Source: CAD feature listing. Evaluate the final solid. Frame: model axes, mm. Give positions to 0.01 mm unless a question says otherwise; leave off trailing zeros. Order: outer loops, then holes, each group sorted by start corner. A loop starts at its lowest first (then second) coordinate and runs counter-clockwise, first axis right, second up.
```python
from build123d import *

# Parameters (mm, degrees)
CYLINDER_R          = 3.4
CYLINDER_DEPTH      = 100
CYLINDER_ROLL_ANGLE = 90
SKETCH_R            = 11
PAD_DEPTH           = 30
SKETCH001_R         = 8.3
POCKET_DEPTH        = 30.001
CHAMFER_SIZE        = 0.5


with BuildPart() as cylinder:
    # Cylinder → Cylinder (new body)
    with BuildSketch(Plane.XY):
        Circle(CYLINDER_R)
    extrude(amount=CYLINDER_DEPTH)


with BuildPart() as cylinder_1:
    # Cylinder roll: moved
    add(cylinder.part.rotate(Axis((0, 0, 0), (1, 0, 0)), CYLINDER_ROLL_ANGLE))


with BuildPart() as cylinder_2:
    # Cylinder placement: moved
    add(cylinder_1.part.moved(Location((0, 16, 8.5))))


with BuildPart() as chamfer_body:
    # Sketch → Pad (new body)
    with BuildSketch(Plane.XY):
        Circle(SKETCH_R)
    extrude(amount=PAD_DEPTH)

    # Sketch001 → Pocket (cut, through all)
    with BuildSketch(Plane(origin=(0, 0, 0), x_dir=(1, 0, 0), z_dir=(0, 0, -1))):
        Circle(SKETCH001_R)
    extrude(amount=-POCKET_DEPTH, mode=Mode.SUBTRACT)

    # Cut: cut Cylinder
    add(cylinder_2.part, mode=Mode.SUBTRACT)

    # Chamfer
    chamfer_edges = [chamfer_body.edges().sort_by_distance(p)[0] for p in [
        (-8.3, 0, 0),
        (-8.3, 0, 30),
        (-11, 0, 30),
    ]]
    chamfer(chamfer_edges, length=CHAMFER_SIZE)


solid = chamfer_body.part
```
1) Section query A-A, the plane x = 0. Return the cut outline in (y, z), and give its area (3 significant figures).
Report:
outline: (-11, 0) - (-8.8, 0) - (-8.3, 0.5) - (-8.3, 5.1) - (-11, 5.1) - close; (-11, 11.9) - (-8.3, 11.9) - (-8.3, 29.5) - (-8.8, 30) - (-10.5, 30) - (-11, 29.5) - close; (8.3, 0.5) - (8.8, 0) - (11, 0) - (11, 5.1) - (8.3, 5.1) - close; (8.3, 11.9) - (11, 11.9) - (11, 29.5) - (10.5, 30) - (8.8, 30) - (8.3, 29.5) - close
area: 125 mm2
2) Section query D-D, the plane z = 15. Return the cut outline in (x, y).
Report:
outline: circle Ø22 at (0, 0); hole circle Ø16.6 at (0, 0)
3) Pin query (flat end, axial travel): pin 1 (1.5 mm diameter, centred on x = -1.5, z = 4, fed in from +Y); pin 2 (6 mm diameter, centred on x = 0, y = -3.5, fed in from -Z); pin 3 (1.5 mm diameter, centred on y = -1, z = 17, fed in from -X); pin 4 (6 mm diameter, centred on x = 5.5, z = 4, fed in from -Y). Return the tip coordinate at first contact, or that it passes through.
Report:
pin 1: stops at y = 10.97
pin 2: passes through
pin 3: stops at x = -11
pin 4: stops at y = -10.71
4) Section query C-C, the plane z = 11.5. Return the cut outline in (x, y).
Report:
outline: (-1.6, -10.88) - (-1.6, -8.14) arc R8.3 cw to (-1.6, 8.14) - (-1.6, 10.88) arc R11 ccw to start; (1.6, -10.88) arc R11 ccw to (1.6, 10.88) - (1.6, 8.14) arc R8.3 cw to (1.6, -8.14) - close
5) Draft query along Y for faces 1 (the cylindrical face through (3.83, 7.364, 14.797)), 2 (the flat face through (0, 9, 0)), 3 (the cylindrical face through (5.076, -9.759, 14.544)). Return one class per face: +Y half, -Y half, draft (parallel to the pull), parting line (faces both ways), or undercut.
Report:
face 1: undercut
face 2: draft
face 3: parting line
6) Material intervals for L1, parallel to Y at x = 0, z = 23; L2, parallel to Z at x = 0, y = -9.75; L3, parallel to Y at x = 1, z = 13, sorted ascending.
Report:
L1: y = -11 to -8.3, 8.3 to 11
L2: z = 0 to 5.1, 11.9 to 30
L3: y = -10.95 to -8.24, 8.24 to 10.95
7) Section query B-B, the plane y = 0. Return the cut outline in (x, z), and give its area (3 significant figures).
Report:
outline: (-11, 0) - (-8.8, 0) - (-8.3, 0.5) - (-8.3, 29.5) - (-8.8, 30) - (-10.5, 30) - (-11, 29.5) - close; (8.3, 0.5) - (8.8, 0) - (11, 0) - (11, 29.5) - (10.5, 30) - (8.8, 30) - (8.3, 29.5) - close
area: 161 mm2
